Part model, mm, in its own coordinate system. A direction names the side the tool comes from. Round coordinates to 2 decimals unless told otherwise and drop trailing zeros. Write each loop counter-clockwise with the first axis right and the second up, starting at its lowest first coordinate (ties: lowest second). Pieces come first, ordered by that corner, then holes. Notation, with made-up numbers: M 5,31.5 L 52,31.5 A12 cw 52,44.5 Z; hole C 52,42.25 d3. An arc over 180 degrees is marked long. Answer as a JSON object with one key per item and string values. Group by question number.
1. Which spindle directions (+Z, -Z, +X, -X, +Y, -Y) get a long thin tool onto all of the face, cutting with end or side? Do faces 4 (the face through (30, 45.1, 19.5)), 5 (the face through (112.4, 110, 20)), 6 (the face through (117, 117.4, 17)), 7 (the face through (35, 55, 18)). Say none if no direction does.
2. Band-saw the part on C-C, the plane z = 7.5. Write the cut outline in (x, y), plus the area to 3 significant figures.
3. Band-saw the part on B-B, the plane y = 45. Write the cut outline in (x, z), plus the area to 3 significant figures.
4. Two-plate mould, pull along Y, no slides. Class faces 1 (the face through (142.513, 19.845, 5.07)), 2 (the face through (75, 0, 5)), 3 (the face through (112.4, 45.1, 19.5)): +Y half, -Y half, draft (parallel to the pull), parting line (faces both ways), or undercut.
5. Drill centre lines: line 1 (Y direction, x = 119.5, z = 25); line 2 (X direction, y = 134.94, z = 3). Where is each one in solid material? Low to high. Write a range as from..to.
6. Band-saw the part on A-A, the plane x = 134.94. Write the cut outline in (y, z), plus the area to 3 significant figures.
7. Drop flat-ended pins along their axis: pin 1 (16 mm diameter, centred on y = 45, z = 25, fed in from -X); pin 2 (3 mm diameter, centred on x = 119.5, z = 20.5, fed in from +Y); pin 3 (10 mm diameter, centred on y = 62, z = 17, fed in from +X); pin 4 (3 mm diameter, centred on x = 34, z = 16.5, fed in from -Y). Give the stop position or say it passes through.
from build123d import *

# Parameters (mm, degrees)
CROQUIS1_W              = 152.4
CROQUIS1_H              = 152.4
SALIENTE_EXTRUIR1_DEPTH = 10
CROQUIS2_R              = 7.94
CORTAR_EXTRUIR1_DEPTH   = 216.758012597
CROQUIS4_R              = 5
SALIENTE_EXTRUIR2_DEPTH = 10


with BuildPart() as part:
    # Croquis1 → Saliente-Extruir1 (new body)
    with BuildSketch(Plane.XY):
        with Locations((76.2, 76.2)):
            Rectangle(CROQUIS1_W, CROQUIS1_H)
    extrude(amount=SALIENTE_EXTRUIR1_DEPTH)

    # Croquis2 → Cortar-Extruir1 (cut, through all)
    with BuildSketch(Plane.XY.offset(10)):
        with Locations((134.94, 17.46)):
            Circle(CROQUIS2_R)
        with Locations((17.46, 17.46)):
            Circle(CROQUIS2_R)
        with Locations(Location((134.94, 134.94, 0), (0, 0, 180))):
            Circle(CROQUIS2_R)
        with Locations(Location((17.46, 134.94, 0), (0, 0, 180))):
            Circle(CROQUIS2_R)
    extrude(amount=-CORTAR_EXTRUIR1_DEPTH, mode=Mode.SUBTRACT)

    # Croquis4 → Saliente-Extruir2 (add)
    # profile 1 of 2: a face of its own
    with BuildSketch(Plane.ZY.offset(-40)):
        with BuildLine():
            Line((10, 117.4), (25, 117.4))
            ThreePointArc((25, 117.4), (35, 107.4), (25, 97.4))
            Line((25, 97.4), (10, 97.4))
            Line((10, 97.4), (10, 117.4))
        make_face()
        with Locations((25, 107.4)):
            Circle(CROQUIS4_R, mode=Mode.SUBTRACT)
    # profile 2 of 2: a face of its own
    with BuildSketch(Plane.ZY.offset(-40)):
        with BuildLine():
            Line((25, 55), (10, 55))
            Line((10, 55), (10, 35))
            Line((10, 35), (25, 35))
            ThreePointArc((25, 35), (35, 45), (25, 55))
        make_face()
        with Locations(Location((25, 45, 0), (0, 0, 180))):
            Circle(CROQUIS4_R, mode=Mode.SUBTRACT)
    saliente_extruir2 = extrude(amount=SALIENTE_EXTRUIR2_DEPTH)

    # Simetría1: Saliente-Extruir2 across plane
    add(saliente_extruir2.mirror(Plane.ZY.offset(-76.2)))


solid = part.part
Worked answers:
{
 "1": {"face 4": "+Z, -X, +Y, -Y", "face 5": "+Z, +Y, -Y", "face 6": "+Z, +X, -X, +Y", "face 7": "+Z, +X, -X"},
 "2": {"outline": "M 0,0 L 152.4,0 L 152.4,152.4 L 0,152.4 Z; hole C 17.46,17.46 d15.88; hole C 17.46,134.94 d15.88; hole C 134.94,17.46 d15.88; hole C 134.94,134.94 d15.88", "area": "22,400 mm^2"},
 "3": {"outline": "M 0,0 L 152.4,0 L 152.4,10 L 122.4,10 L 122.4,20 L 112.4,20 L 112.4,10 L 40,10 L 40,20 L 30,20 L 30,10 L 0,10 Z; M 30,30 L 40,30 L 40,35 L 30,35 Z; M 112.4,30 L 122.4,30 L 122.4,35 L 112.4,35 Z", "area": "1,820 mm^2"},
 "4": {"face 1": "undercut", "face 2": "-Y half", "face 3": "draft"},
 "5": {"line 1": "y = 35..40, 50..55, 97.4..102.4, 112.4..117.4", "line 2": "x = 0..9.52, 25.4..127, 142.88..152.4"},
 "6": {"outline": "M 0,0 L 9.52,0 L 9.52,10 L 0,10 Z; M 25.4,0 L 127,0 L 127,10 L 25.4,10 Z; M 142.88,0 L 152.4,0 L 152.4,10 L 142.88,10 Z", "area": "1,210 mm^2"},
 "7": {"pin 1": "stops at x = 30", "pin 2": "stops at y = 117.4", "pin 3": "passes through", "pin 4": "stops at y = 35"}
}
